Geometry check sheet. Reference: the model listing, model coordinates, mm. A direction names the side the tool comes from. Round coordinates to 2 decimals unless told otherwise and drop trailing zeros. Write each loop counter-clockwise with the first axis right and the second up, starting at its lowest first coordinate (ties: lowest second). Pieces come first, ordered by that corner, then holes. Notation, with made-up numbers: (-39.5, 77) - (-27.5, 77) arc R29 ccw to (-27.5, 104) - close; hole circle Ø1 at (-11, -37.5). An arc over 180 degrees is marked (long way). Return JSON: item names as keys, results as strings. Group by question number.
from build123d import *

# Parameters (mm, degrees)
F0_R     = 3.975
F0_R_2   = 3
F1_DEPTH = 15
F4_DEPTH = 3


with BuildPart() as f1:
    # F0 (on Front) → F1 (new body)
    with BuildSketch(Plane.XZ):
        Circle(F0_R)
        Circle(F0_R_2, mode=Mode.SUBTRACT)
    extrude(amount=F1_DEPTH)

    # F3 (on offset) → F4 (cut)
    with BuildSketch(Plane.YZ.offset(3.975)):
        with BuildLine():
            Line((-15, 2), (-15, -2))
            Line((-15, -2), (-13, -2))
            ThreePointArc((-13, -2), (-11, 0), (-13, 2))
            Line((-13, 2), (-15, 2))
        make_face()
    extrude(amount=-F4_DEPTH, mode=Mode.SUBTRACT)


solid = f1.part
1. Material ranges on line 1 along Z through (x, y) = (0, -6.25) (3 decimals); line 2 along Z through (x, y) = (-2.5, -3), recorded low to high.
2. Section check D-D (x = -3.25). Enter the section's corners in (y, z).
3. Section check B-B (x = -1.75). Enter the section's corners in (y, z).
4. Section check C-C (y = -0.75). Enter the section's corners in (x, z) (3 decimals), and give its area (3 significant figures).
5. Mould release check, pull along X, two halves, no side actions. Record for faces 1 (the face through (3, -14, 2)), 2 (the face through (-3, -7, 0)), 3 (the face through (-3.97, -7.4, 0.17)): pulls with the +X half, pulls with the -X half, needs draft (parallel to the pull), parting line crosses it, or undercut.
6. Depth check by flat-ended pin: pin 1 Ø2 at (y, z) = (-3, -2.5) entering from +X; pin 2 Ø1.3 at (x, y) = (3, -13.5) entering from -Z; pin 3 Ø1.5 at (y, z) = (-8, -1.5) entering from +X. Enter the tip coordinate at first touch or a pass-through.
7. Tool access check on faces 4 (the face through (3, -14, -2)), 5 (the face through (-3, -15, 1)). Record the directions out of +Z, -Z, +X, -X, +Y, -Y that give a thin tool (end or side, any length) a straight path to the whole face; none if there is none.
8. Section check A-A (z = 0). Enter the section's corners in (x, y) (3 decimals).
Result sheet:
{
 "1": {"line 1": "z = -3.975 to -3, 3 to 3.975", "line 2": "z = -3.09 to -1.66, 1.66 to 3.09"},
 "2": {"outline": "(-15, -2.29) - (0, -2.29) - (0, 2.29) - (-15, 2.29) - close"},
 "3": {"outline": "(-15, -3.57) - (0, -3.57) - (0, -2.44) - (-15, -2.44) - close; (-15, 2.44) - (0, 2.44) - (0, 3.57) - (-15, 3.57) - close"},
 "4": {"outline": "circle Ø7.95 at (0, 0); hole circle Ø6 at (0, 0)", "area": "21.4 mm²"},
 "5": {"face 1": "needs draft", "face 2": "undercut", "face 3": "parting line crosses it"},
 "6": {"pin 1": "stops at x = 3.68", "pin 2": "stops at z = -3.21", "pin 3": "stops at x = 3.9"},
 "7": {"face 4": "+X, -Y", "face 5": "+Z, -Z, +X, -X, -Y"},
 "8": {"outline": "(-3.975, -15) - (-3, -15) - (-3, 0) - (-3.975, 0) - close; (3, -11) - (3.975, -11) - (3.975, 0) - (3, 0) - close"}
}
